from build123d import *

# Parameters (mm, degrees)
EXTRUDE015_DEPTH = 1
EXTRUDE014_DEPTH = 2.75


with BuildPart() as extrude015:
    # Sketch015 → Extrude015 (new body)
    with BuildSketch(Plane.XZ):
        with BuildLine():
            ThreePointArc((11.7, 16.35), (11.063604, 16.086396), (10.8, 15.45))
            Line((10.8, 14.2), (10.8, 15.45))
            ThreePointArc((10.8, 14.2), (11.23934, 13.13934), (12.3, 12.7))
            Line((16.8, 12.7), (12.3, 12.7))
            ThreePointArc((16.8, 12.7), (17.86066, 13.13934), (18.3, 14.2))
            Line((18.3, 15.45), (18.3, 14.2))
            ThreePointArc((18.3, 15.45), (18.036396, 16.086396), (17.4, 16.35))
            Line((11.7, 16.35), (17.4, 16.35))
        make_face()
    extrude(amount=EXTRUDE015_DEPTH)


with BuildPart() as extrude015_1:
    # Extrude015 placement: moved
    add(extrude015.part.moved(Location((0, 2.5, 0))))


with BuildPart() as button1:
    # Sketch014 → Extrude014 (new body)
    with BuildSketch(Plane.XZ):
        with BuildLine():
            ThreePointArc((12.75, 16.13), (12.113604, 15.866396), (11.85, 15.23))
            Line((11.85, 14.43), (11.85, 15.23))
            ThreePointArc((11.85, 14.43), (12.113604, 13.793604), (12.75, 13.53))
            Line((16.35, 13.53), (12.75, 13.53))
            ThreePointArc((16.35, 13.53), (16.986396, 13.793604), (17.25, 14.43))
            Line((17.25, 15.23), (17.25, 14.43))
            ThreePointArc((17.25, 15.23), (16.986396, 15.866396), (16.35, 16.13))
            Line((12.75, 16.13), (16.35, 16.13))
        make_face()
    extrude(amount=EXTRUDE014_DEPTH)


with BuildPart() as button1_1:
    # Extrude014 placement: moved
    add(button1.part.moved(Location((0, 2, 0))))

    # Fusion018: union Extrude015
    add(extrude015_1.part)


solid = button1_1.part
For this review, take the finished solid that the model builds, in its own axes (mm). A direction names the side the tool comes from. Round coordinates to 2 decimals unless told otherwise and drop trailing zeros. Loops run counter-clockwise (first coordinate to the right, second up) from the corner with the lowest first, then second, coordinate; pieces in that order, holes last. Notation, with made-up numbers: (31.25, -37.5) - (75.25, -37.5) arc R19 cw to (75.25, -17.5) - close; hole circle Ø7 at (60, 75.25). An arc over 180 degrees is marked (long way). Answer as CSV lines item,"result".
(1) Insertion check: P1, Ø1.1, axis at x = 15, y = 0, coming from the -Z side; P2, Ø0.6, axis at y = 0, z = 14.5, coming from the +X side; P3, Ø1, axis at x = 16.5, y = 0.5, coming from the +Z side. Each pin has a flat end and moves straight along its axis. Give the tip position at first contact, or say it passes through.
Checked values:
P1,"stops at z = 13.53"
P2,"stops at x = 17.25"
P3,"stops at z = 16.13"
(2) Tool access review of faces 1 (the face through (11.85, 0, 15)), 2 (the face through (12.12, 0.39, 15.87)), 3 (the face through (16.99, 0.39, 15.86)), 4 (the face through (16.98, 0.39, 13.79)): name each direction out of +Z, -Z, +X, -X, +Y, -Y from which nothing blocks a thin tool from reaching the whole face with its end or side.
Checked values:
face 1,"+Z, -Z, -X, -Y"
face 2,"+Z, -X, -Y"
face 3,"+Z, +X, -Y"
face 4,"-Z, +X, -Y"
(3) Consider section A-A on y = -0.1. Give the boundary of the cut face in (x, z).
Checked values:
outline,"(11.85, 14.43) arc R0.9 ccw to (12.75, 13.53) - (16.35, 13.53) arc R0.9 ccw to (17.25, 14.43) - (17.25, 15.23) arc R0.9 ccw to (16.35, 16.13) - (12.75, 16.13) arc R0.9 ccw to (11.85, 15.23) - close"
(4) Wall thickness on line 1 (X direction, y = -0.45, z = 14.55); line 2 (Z direction, x = 14.75, y = -0.6); line 3 (Y direction, x = 15, z = 13.2): over which ranges is each line inside the solid? List them lowest first.
Checked values:
line 1,"x = 11.85 to 17.25"
line 2,"z = 13.53 to 16.13"
line 3,"y = 1.5 to 2.5"
(5) Consider section C-C on z = 13.2. Give the boundary of the cut face in (x, y), then the cut area to 3 significant figures.
Checked values:
outline,"(11.18, 1.5) - (17.92, 1.5) - (17.92, 2.5) - (11.18, 2.5) - close"
area,"6.74 mm2"
(6) Consider section B-B on x = 14. Give the boundary of the cut face in (y, z), then the cut area to 3 significant figures.
Checked values:
outline,"(-0.75, 13.53) - (1.5, 13.53) - (1.5, 12.7) - (2.5, 12.7) - (2.5, 16.35) - (1.5, 16.35) - (1.5, 16.13) - (-0.75, 16.13) - close"
area,"9.50 mm2"
